```python
from build123d import *

# Parameters (mm, degrees)
SKETCH1_W           = 220
SKETCH1_H           = 70
BOSS_EXTRUDE1_DEPTH = 3
SKETCH2_2_R         = 1.5
CUT_EXTRUDE2_DEPTH  = 231.887418453
SKETCH3_W           = 3
SKETCH3_H           = 20
BOSS_EXTRUDE4_DEPTH = 3
LPATTERN1_COUNT     = 2
LPATTERN1_PITCH     = 25
LPATTERN1_COL_COUNT = 2
LPATTERN1_COL_PITCH = 25
SKETCH4_W           = 30
SKETCH4_H           = 3
CUT_EXTRUDE3_DEPTH  = 234.747727262
SKETCH5_R           = 5.5
CUT_EXTRUDE4_DEPTH  = 234.747727262
SKETCH6_W           = 13
SKETCH6_H           = 5
CUT_EXTRUDE5_DEPTH  = 234.747727262


with BuildPart() as part:
    # Sketch1 → Boss-Extrude1 (new body)
    with BuildSketch(Plane.XY):
        with Locations((110, 35)):
            Rectangle(SKETCH1_W, SKETCH1_H)
    extrude(amount=BOSS_EXTRUDE1_DEPTH)

    # Sketch2<2> → Cut-Extrude2 (cut, through all)
    with BuildSketch(Plane.XY.offset(3)):
        with Locations((5, 65)):
            Circle(SKETCH2_2_R)
        with Locations((5, 5)):
            Circle(SKETCH2_2_R)
        with Locations((215, 5)):
            Circle(SKETCH2_2_R)
        with Locations((215, 65)):
            Circle(SKETCH2_2_R)
    extrude(amount=-CUT_EXTRUDE2_DEPTH, mode=Mode.SUBTRACT)

    # Sketch3 → Boss-Extrude4 (add)
    with BuildSketch(Plane.XY.offset(3)):
        with Locations((-1.5, 35)):
            Rectangle(SKETCH3_W, SKETCH3_H)
        with Locations((221.5, 35)):
            Rectangle(SKETCH3_W, SKETCH3_H)
    boss_extrude4 = extrude(amount=-BOSS_EXTRUDE4_DEPTH)

    # LPattern1: Boss-Extrude4 ×2
    with Locations(*[(0, i * LPATTERN1_PITCH, 0) for i in range(1, LPATTERN1_COUNT)]):
        add(boss_extrude4)

    # LPattern1 col: Boss-Extrude4 ×2
    with Locations(*[(0, -i * LPATTERN1_COL_PITCH, 0) for i in range(1, LPATTERN1_COL_COUNT)]):
        add(boss_extrude4)

    # Sketch4 → Cut-Extrude3 (cut, through all)
    with BuildSketch(Plane(origin=(0, 0, 0), x_dir=(-1, 0, 0), z_dir=(0, 0, -1))):
        with Locations((-170, 1.5)):
            Rectangle(SKETCH4_W, SKETCH4_H)
        with Locations((-110, 1.5)):
            Rectangle(SKETCH4_W, SKETCH4_H)
        with Locations((-50, 1.5)):
            Rectangle(SKETCH4_W, SKETCH4_H)
    extrude(amount=-CUT_EXTRUDE3_DEPTH, mode=Mode.SUBTRACT)

    # Sketch5 → Cut-Extrude4 (cut, through all)
    with BuildSketch(Plane.XY.offset(3)):
        with Locations((158, 29)):
            Circle(SKETCH5_R)
    extrude(amount=-CUT_EXTRUDE4_DEPTH, mode=Mode.SUBTRACT)

    # Sketch6 → Cut-Extrude5 (cut, through all)
    with BuildSketch(Plane(origin=(0, 0, 0), x_dir=(-1, 0, 0), z_dir=(0, 0, -1))):
        with Locations((-140, 48)):
            Rectangle(SKETCH6_W, SKETCH6_H)
        with Locations((-190, 48)):
            Rectangle(SKETCH6_W, SKETCH6_H)
        with Locations((-190, 38)):
            Rectangle(SKETCH6_W, SKETCH6_H)
        with Locations((-190, 28)):
            Rectangle(SKETCH6_W, SKETCH6_H)
        with Locations((-190, 18)):
            Rectangle(SKETCH6_W, SKETCH6_H)
        with Locations((-140, 38)):
            Rectangle(SKETCH6_W, SKETCH6_H)
        with Locations((-140, 28)):
            Rectangle(SKETCH6_W, SKETCH6_H)
        with Locations((-140, 18)):
            Rectangle(SKETCH6_W, SKETCH6_H)
        with Locations((-80, 18)):
            Rectangle(SKETCH6_W, SKETCH6_H)
        with Locations((-80, 28)):
            Rectangle(SKETCH6_W, SKETCH6_H)
        with Locations((-80, 38)):
            Rectangle(SKETCH6_W, SKETCH6_H)
        with Locations((-30, 18)):
            Rectangle(SKETCH6_W, SKETCH6_H)
        with Locations((-30, 28)):
            Rectangle(SKETCH6_W, SKETCH6_H)
        with Locations((-30, 38)):
            Rectangle(SKETCH6_W, SKETCH6_H)
        with Locations((-30, 48)):
            Rectangle(SKETCH6_W, SKETCH6_H)
        with Locations((-80, 48)):
            Rectangle(SKETCH6_W, SKETCH6_H)
    extrude(amount=-CUT_EXTRUDE5_DEPTH, mode=Mode.SUBTRACT)


solid = part.part
```
The listing builds one solid part. Answer for the finished solid, in the listing's coordinates (mm). Round coordinates to 2 decimals unless told otherwise and drop trailing zeros. Order: outer loops, then holes, each group sorted by start corner. A loop starts at its lowest first (then second) coordinate and runs counter-clockwise, first axis right, second up. Notation, with made-up numbers: (6.5, 59.25) -> (56.5, 59.25) arc R13 ccw to (56.5, 74.25) -> close; hole circle Ø4 at (-22, -1.5). An arc over 180 degrees is marked (long way). Answer as CSV lines item,"result". Start each with the question number.
(1) Find the intervals of material crossed by probe 1 along Y at (x, z) = (194, 1.1); probe 2 along Y at (x, z) = (215, 1.55); probe 3 along X at (y, z) = (65, 1.85), in increasing order. Write a range as from..to.
(2) The part is cut by section A-A (x = 144.5). Determine the outline of the cut face in (y, z), then the cut area to 3 significant figures.
(3) For a pull along X with two mould halves and no side action, classify faces 1 (the face through (108, 35, 3)), 2 (the face through (152.505, 29.242, 1.521)) as +X half, -X half, draft (parallel to the pull), parting line (faces both ways), or undercut.
(4) The part is cut by section B-B (x = 174). Determine the outline of the cut face in (y, z), then the cut area to 3 significant figures.
(5) A flat-ended cylindrical pin translates along its axis: pin 1 Ø1.5 at (y, z) = (47, 1.5) entering from +X. Find the tip coordinate at first contact, or state that the pin passes through.
(6) The part is cut by section C-C (z = 0.5). Count the separate pieces of the cut face and the enclosed holes in it, then the cut area to 3 significant figures.
Evaluation:
1,probe 1,"0..15.5, 20.5..25.5, 30.5..35.5, 40.5..45.5, 50.5..70"
1,probe 2,"0..3.5, 6.5..63.5, 66.5..70"
1,probe 3,"-3..3.5, 6.5..213.5, 216.5..223"
2,outline,"(0, 0) -> (15.5, 0) -> (15.5, 3) -> (0, 3) -> close; (20.5, 0) -> (25.5, 0) -> (25.5, 3) -> (20.5, 3) -> close; (30.5, 0) -> (35.5, 0) -> (35.5, 3) -> (30.5, 3) -> close; (40.5, 0) -> (45.5, 0) -> (45.5, 3) -> (40.5, 3) -> close; (50.5, 0) -> (70, 0) -> (70, 3) -> (50.5, 3) -> close"
2,area,"150 mm²"
3,face 1,"draft"
3,face 2,"undercut"
4,outline,"(3, 0) -> (70, 0) -> (70, 3) -> (3, 3) -> close"
4,area,"201 mm²"
5,pin 1,"x = 220"
6,separate pieces,"1"
6,enclosed holes,"21"
6,area,"14,300 mm²"
